Autodesk Inventor part; units mm, degrees
ref_plane "YZ Plane" through (0, 0, 0) normal (1, 0, 0) x (0, 1, 0)
ref_plane "XZ Plane" through (0, 0, 0) normal (0, 1, 0) x (-1, 0, 0)
ref_plane "XY Plane" through (0, 0, 0) normal (0, 0, 1) x (1, 0, 0)
sketch "Sketch1" plane through (0, 0, 0) normal (0, 0, 1) x (1, 0, 0)
  line L0 (-17, 4) -> (43, 4) construction
  line L1 (-17, -1) -> (43, -1)
  line L2 (43, 9) -> (-17, 9)
  arc A0 (-17, 9) -> (-17, -1) centre (-17, 4) ccw
  arc A1 (43, -1) -> (43, 9) centre (43, 4) ccw
  circle A2 centre (-17, 4) radius 2.5
  circle A3 centre (43, 4) radius 2.5
  point P0 (0, 0)
  point P1 (13, 4)
  dimension "d0" = 60
  dimension "d1" = 10
  dimension "d2" = 5
extrude "Extrusion1" add sketch "Sketch1" along normal blind 5 contours A0 L2 A1 L1 | A2
extrude "Extrusion2" add sketch "Sketch1" against normal blind 5 contours A2
Could you check a few things on this model? Use its own coordinates, in mm. Give positions to 0.01 mm unless a question says otherwise; leave off trailing zeros. Order: outer loops, then holes, each group sorted by start corner. A loop starts at its lowest first (then second) coordinate and runs counter-clockwise, first axis right, second up.
Item 1: I'm going to push flat-ended pins straight in: pin 1 (6 mm diameter, centred on x = 25, y = 3, fed in from -Z); pin 2 (4 mm diameter, centred on x = 26.5, z = -1, fed in from +Y). Where does each tip first touch, or does it pass through?
Item 2: If we section it at C-C, the plane z = 2.75: Write out the boundary of the cut face in (x, y), plus the area to 3 significant figures.
Item 3: If we section it at D-D, the plane z = -1.25: Write out the boundary of the cut face in (x, y).
Item 4: If we section it at A-A, the plane y = 4: Write out the boundary of the cut face in (x, z).
Item 5: If we mould it in two halves opening along Y, with no side actions, what happens to faces 1 (the face through (13, -1, 2)), 2 (the face through (45.385, 3.249, 2.465)), 3 (the face through (-19.5, 4.1, -2.5)), 4 (the face through (13, 4, 0))? For each: pulls with the +Y half, pulls with the -Y half, needs draft (parallel to the pull), parting line crosses it, or undercut.
Item 6: If we section it at B-B, the plane x = -18: Write out the boundary of the cut face in (y, z), plus the area to 3 significant figures.
Item 7: I need wall thicknesses on line 1 (Y direction, x = 43, z = 1.25); line 2 (Z direction, x = 1, y = 7.25); line 3 (X direction, y = 5, z = 1.5). Which ranges of each line are inside material? Lowest first, please.
Values:
1. pin 1: stops at z = 0
1. pin 2: stops at y = 9
2. outline: (-17, -1) - (43, -1) arc R5 ccw to (43, 9) - (-17, 9) arc R5 ccw to start; hole circle Ø5 at (43, 4)
2. area: 659 mm2
3. outline: circle Ø5 at (-17, 4)
4. outline: (-22, 0) - (-19.5, 0) - (-19.5, -5) - (-14.5, -5) - (-14.5, 0) - (40.5, 0) - (40.5, 5) - (-22, 5) - close; (45.5, 0) - (48, 0) - (48, 5) - (45.5, 5) - close
5. face 1: pulls with the -Y half
5. face 2: undercut
5. face 3: parting line crosses it
5. face 4: needs draft
6. outline: (-0.9, 0) - (1.71, 0) - (1.71, -5) - (6.29, -5) - (6.29, 0) - (8.9, 0) - (8.9, 5) - (-0.9, 5) - close
6. area: 71.9 mm2
7. line 1: y = -1 to 1.5, 6.5 to 9
7. line 2: z = 0 to 5
7. line 3: x = -21.9 to 40.71, 45.29 to 47.9
